from build123d import *

# Parameters (mm, degrees)
SKETCH1_W                   = 76.2
SKETCH1_H                   = 19.05
BOSS_EXTRUDE1_DEPTH         = 5.588
F_1_4_CLEARANCE_HOLE1_D     = 6.7564
F_1_4_CLEARANCE_HOLE1_DEPTH = 19.05
F_1_4_CLEARANCE_HOLE1_TIP   = 2.029827343
F_6_CLEARANCE_HOLE1_D       = 3.5052


with BuildPart() as part:
    # Sketch1 → Boss-Extrude1 (new body)
    with BuildSketch(Plane(origin=(0, 0, 0), x_dir=(1, 0, 0), z_dir=(0, 1, 0))):
        Rectangle(SKETCH1_W, SKETCH1_H)
    extrude(amount=BOSS_EXTRUDE1_DEPTH)

    # 1/4 Clearance Hole1
    with Locations(Plane(origin=(0, 5.588, 0), x_dir=(1, 0, 0), z_dir=(0, 1, 0))):
        with Locations((0, 0)):
            Hole(F_1_4_CLEARANCE_HOLE1_D / 2, depth=F_1_4_CLEARANCE_HOLE1_DEPTH)
            with Locations((0, 0, -(F_1_4_CLEARANCE_HOLE1_DEPTH + F_1_4_CLEARANCE_HOLE1_TIP / 2))):  # 118° drill point
                Cone(0, F_1_4_CLEARANCE_HOLE1_D / 2, F_1_4_CLEARANCE_HOLE1_TIP, mode=Mode.SUBTRACT)

    # #6 Clearance Hole1 (through all)
    with Locations(Plane(origin=(0, 5.588, 0), x_dir=(1, 0, 0), z_dir=(0, 1, 0))):
        with Locations((25.4, 0), (-25.4, 0)):
            Hole(F_6_CLEARANCE_HOLE1_D / 2)


solid = part.part
Here's how the part is built. I have some questions about the finished solid (model axes, mm). Round coordinates to 2 decimals unless told otherwise and drop trailing zeros. Write each loop counter-clockwise with the first axis right and the second up, starting at its lowest first coordinate (ties: lowest second). Pieces come first, ordered by that corner, then holes.
1. Suppose I cut it at A-A (x = 25.4). List the corners of the cut face in (y, z) for me (3 decimals), and give its area (3 significant figures).
2. Suppose I cut it at C-C (y = 3.25). List the corners of the cut face in (x, z) for me (3 decimals).
3. Suppose I cut it at D-D (x = 0). List the corners of the cut face in (y, z) for me (3 decimals).
4. Suppose I cut it at B-B (z = 0). List the corners of the cut face in (x, y) for me, and give its area (3 significant figures).
5. If we mould it in two halves opening along Z, with no side actions, what happens to faces 1 (the cylindrical face through (26.692, 2.755, -1.184)), 2 (the flat face through (-1, 3, 9.525)), 3 (the cylindrical face through (-27.07, 2.75, -0.53)), 4 (the flat face through (-1, 0, -4))? For each: released by +Z, released by -Z, zero draft, split by the parting line, or undercut.
6. I need wall thicknesses on L1, parallel to X at y = 0.85, z = -0.75; L2, parallel to Z at x = 25.4, y = 2.1 (3 decimals); L3, parallel to Z at x = 0, y = 3.05 (3 decimals). Which ranges of each line are inside material? Lowest first, please.
Answer sheet:
1. outline: (0, -9.525) - (5.588, -9.525) - (5.588, -1.753) - (0, -1.753) - close; (0, 1.753) - (5.588, 1.753) - (5.588, 9.525) - (0, 9.525) - close
1. area: 86.9 mm2
2. outline: (-38.1, -9.525) - (38.1, -9.525) - (38.1, 9.525) - (-38.1, 9.525) - close; hole circle Ø3.505 at (-25.4, 0); hole circle Ø6.756 at (0, 0); hole circle Ø3.505 at (25.4, 0)
3. outline: (0, -9.525) - (5.588, -9.525) - (5.588, -3.378) - (0, -3.378) - close; (0, 3.378) - (5.588, 3.378) - (5.588, 9.525) - (0, 9.525) - close
4. outline: (-38.1, 0) - (-27.15, 0) - (-27.15, 5.59) - (-38.1, 5.59) - close; (-23.65, 0) - (-3.38, 0) - (-3.38, 5.59) - (-23.65, 5.59) - close; (3.38, 0) - (23.65, 0) - (23.65, 5.59) - (3.38, 5.59) - close; (27.15, 0) - (38.1, 0) - (38.1, 5.59) - (27.15, 5.59) - close
4. area: 349 mm2
5. face 1: undercut
5. face 2: released by +Z
5. face 3: undercut
5. face 4: zero draft
6. L1: x = -38.1 to -26.98, -23.82 to -3.29, 3.29 to 23.82, 26.98 to 38.1
6. L2: z = -9.525 to -1.753, 1.753 to 9.525
6. L3: z = -9.525 to -3.378, 3.378 to 9.525
